```python
from build123d import *

# Parameters (mm, degrees)
CROQUIS1_R              = 15
SALIENTE_EXTRUIR1_DEPTH = 2.5
CROQUIS2_R              = 4.5
SALIENTE_EXTRUIR2_DEPTH = 3
CROQUIS3_R              = 2.75
CORTAR_EXTRUIR1_DEPTH   = 3
CORTAR_EXTRUIR2_REACH   = 23.915
CROQUIS4_R              = 1.9
CORTAR_EXTRUIR4_REACH   = 23.424
CROQUIS6_R              = 1.9
CORTAR_EXTRUIR3_START   = -1.5
CORTAR_EXTRUIR3_DEPTH   = 2.5
MATRIZC1_COUNT          = 4
CORTAR_EXTRUIR5_DEPTH   = 3
MATRIZC2_COUNT          = 14
REDONDEO1_R             = 1
CROQUIS9_R              = 3.2
CORTAR_EXTRUIR6_DEPTH   = 1.5


with BuildPart() as part:
    # Croquis1 → Saliente-Extruir1 (new body)
    with BuildSketch(Plane(origin=(0, 0, 0), x_dir=(1, 0, 0), z_dir=(0, 1, 0))):
        with Locations(Location((0, 0, 0), (0, 0, 270))):
            Circle(CROQUIS1_R)
    extrude(amount=SALIENTE_EXTRUIR1_DEPTH)

    # Croquis2 → Saliente-Extruir2 (add)
    with BuildSketch(Plane(origin=(0, 2.5, 0), x_dir=(1, 0, 0), z_dir=(0, 1, 0))):
        with Locations(Location((0, 0, 0), (0, 0, 270))):
            Circle(CROQUIS2_R)
    extrude(amount=SALIENTE_EXTRUIR2_DEPTH)

    # Croquis3 → Cortar-Extruir1 (cut)
    with BuildSketch(Plane(origin=(0, 5.5, 0), x_dir=(1, 0, 0), z_dir=(0, 1, 0))):
        with Locations(Location((0, 0, 0), (0, 0, 270))):
            Circle(CROQUIS3_R)
    extrude(amount=-CORTAR_EXTRUIR1_DEPTH, mode=Mode.SUBTRACT)

    # Croquis4 → Cortar-Extruir2 (cut, up to next)
    with BuildSketch(Plane.XZ, mode=Mode.PRIVATE) as cortar_extruir2_sk1:
        with Locations(Location((0, 0, 0), (0, 0, 270))):
            Circle(CROQUIS4_R)
    cortar_extruir2_tool1 = extrude(cortar_extruir2_sk1.sketch, amount=-CORTAR_EXTRUIR2_REACH, mode=Mode.PRIVATE) & part.part
    add(cortar_extruir2_tool1.solids().sort_by_distance((0, 0, 0))[0], mode=Mode.SUBTRACT)

    # Croquis6 → Cortar-Extruir4 (cut, up to next)
    with BuildSketch(Plane(origin=(0, 2.5, 0), x_dir=(1, 0, 0), z_dir=(0, 1, 0)), mode=Mode.PRIVATE) as cortar_extruir4_sk1:
        with Locations(Location((0, 10.5, 0), (0, 0, 270))):
            Circle(CROQUIS6_R)
    cortar_extruir4_tool1 = extrude(cortar_extruir4_sk1.sketch, amount=-CORTAR_EXTRUIR4_REACH, mode=Mode.PRIVATE) & part.part
    cortar_extruir4 = cortar_extruir4_tool1.solids().sort_by_distance((0, 2.5, -10.5))[0]
    add(cortar_extruir4, mode=Mode.SUBTRACT)

    # Croquis5 → Cortar-Extruir3 (cut)
    with BuildSketch(Plane(origin=(0, 2.5, 0), x_dir=(1, 0, 0), z_dir=(0, 1, 0)).offset(CORTAR_EXTRUIR3_START)):
        Polygon((-1.818653348, 13.65), (-3.637306696, 10.5), (-1.818653348, 7.35), (1.818653348, 7.35), (3.637306696, 10.5), (1.818653348, 13.65), align=None)
    cortar_extruir3 = extrude(amount=CORTAR_EXTRUIR3_DEPTH, mode=Mode.SUBTRACT)

    # MatrizC1: Cortar-Extruir4, Cortar-Extruir3 ×4 about axis
    matrizc1_axis = Axis((0, 0, 0), (0, 1, 0))
    add([cortar_extruir4.rotate(matrizc1_axis, i * 360 / MATRIZC1_COUNT) for i in range(1, MATRIZC1_COUNT)], mode=Mode.SUBTRACT)
    add([cortar_extruir3.rotate(matrizc1_axis, i * 360 / MATRIZC1_COUNT) for i in range(1, MATRIZC1_COUNT)], mode=Mode.SUBTRACT)

    # Croquis7 → Cortar-Extruir5 (cut)
    with BuildSketch(Plane(origin=(0, 5.5, 0), x_dir=(1, 0, 0), z_dir=(0, 1, 0))):
        with BuildLine():
            Line((0, 3.95), (0.6, 2.68374738))
            ThreePointArc((0.6, 2.68374738), (0, 2.75), (-0.6, 2.68374738))
            Line((-0.6, 2.68374738), (0, 3.95))
        make_face()
    cortar_extruir5 = extrude(amount=-CORTAR_EXTRUIR5_DEPTH, mode=Mode.SUBTRACT)

    # MatrizC2: Cortar-Extruir5 ×14 about axis
    matrizc2_axis = Axis((0, 0, 0), (0, 1, 0))
    for i in range(1, MATRIZC2_COUNT):
        add(cortar_extruir5.rotate(matrizc2_axis, i * 360 / MATRIZC2_COUNT), mode=Mode.SUBTRACT)

    # Redondeo1
    redondeo1_edges = [part.edges().sort_by_distance(p)[0] for p in [
        (0, 2.5, -15),
        (0, 2.5, -4.5),
    ]]
    fillet(redondeo1_edges, radius=REDONDEO1_R)

    # Croquis9 → Cortar-Extruir6 (cut)
    with BuildSketch(Plane.XZ):
        with Locations(Location((0, 0, 0), (0, 0, 270))):
            Circle(CROQUIS9_R)
    extrude(amount=-CORTAR_EXTRUIR6_DEPTH, mode=Mode.SUBTRACT)


solid = part.part
```
CAD build for the part. Positions are in the model's coordinates, mm. A direction names the side the tool comes from. Coordinates: 2 decimals unless noted, no trailing zeros. Order: outer loops, then holes, each group sorted by start corner. A loop starts at its lowest first (then second) coordinate and runs counter-clockwise, first axis right, second up. Notation, with made-up numbers: (-8.5, 5.5) -> (42.5, 5.5) arc R9 ccw to (42.5, 14.5) -> close; hole circle Ø6 at (9, -30). An arc over 180 degrees is marked (long way). Use one line per item in the form item = value. Start each with the question number.
1) Drop flat-ended pins along their axis: pin 1 (0.8 mm diameter, centred on y = 2, z = 0.5, fed in from -X); pin 2 (5 mm diameter, centred on x = 9.5, z = -1.5, fed in from +Y); pin 3 (2.5 mm diameter, centred on x = 0, z = 0, fed in from +Y); pin 4 (6 mm diameter, centred on x = 10.5, z = 0, fed in from +Y). Give the stop position or say it passes through.
2) Pull direction X, two halves, no side cores. Call faces 1 (the cylindrical face through (0.66, 0.74, -14.985)), 2 (the flat face through (-3.177, 4.021, -1.028)), 3 (the flat face through (-6, 2.5, 0)): +X half, -X half, draft (parallel to the pull), parting line (faces both ways), or undercut.
3) Band-saw the part on A-A on y = 0.65. Give the cut face in (x, z), then the cut area to 3 significant figures.
4) Drill centre lines: L1, parallel to X at y = 2.05, z = 0; L2, parallel to Z at x = -1.5, y = 2.1; L3, parallel to Y at x = 11.25, z = 6.75. Where is each one in solid material? Low to high. Write a range as [from, to].
5) Tool access for faces 4 (the flat face through (-3, 5.5, 0)), 5 (the flat face through (7.35, 2, 0)): list every direction of +Z, -Z, +X, -X, +Y, -Y with a clear straight run to the whole face (end or side of a thin tool).
Entries:
q1.pin_1 = -14.99
q1.pin_2 = 2.5
q1.pin_3 = through
q1.pin_4 = 1
q2.face_1 = parting line
q2.face_2 = undercut
q2.face_3 = draft
q3.outline = circle Ø30 at (0, 0); hole circle Ø3.8 at (-10.5, 0); hole circle Ø6.4 at (0, 0); hole circle Ø3.8 at (0, -10.5); hole circle Ø3.8 at (0, 10.5); hole circle Ø3.8 at (10.5, 0)
q3.area = 629 mm2
q4.L1 = [-14.84, -13.65], [-7.35, -1.9], [1.9, 7.35], [13.65, 14.84]
q4.L2 = [-14.72, -13.65], [-7.35, -1.17], [1.17, 7.35], [13.65, 14.72]
q4.L3 = [0, 2.5]
q5.face_4 = +Z, -Z, +X, -X, +Y
q5.face_5 = +Y
